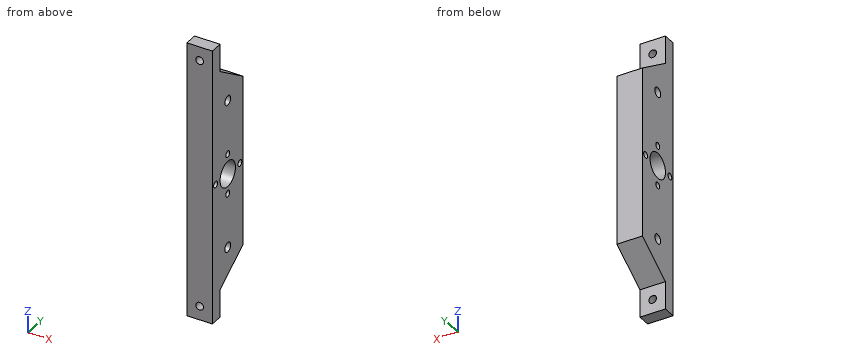
```python
from build123d import *

# Parameters (mm, degrees)
SKETCH2_W               = 380
SKETCH2_H               = 40
SKETCH2_R               = 10
SKETCH2_R_2             = 3.75
BOSS_EXTRUDE2_DEPTH     = 20
CUT_EXTRUDE1_DEPTH      = 100
CUT_EXTRUDE2_DEPTH      = 301.779846116
CUT_EXTRUDE2_DEPTH_BACK = 301.779846116
SKETCH5_R               = 3.023423491
SKETCH8_R               = 2.5
CUT_EXTRUDE3_DEPTH      = 302.941245658


with BuildPart() as part:
    # Sketch2 → Boss-Extrude2 (new body)
    with BuildSketch(Plane(origin=(0, 0, 0), x_dir=(0, 0, -1), z_dir=(1, 0, 0))):
        with Locations((190, 20)):
            Rectangle(SKETCH2_W, SKETCH2_H)
        with Locations((190, 20)):
            Circle(SKETCH2_R, mode=Mode.SUBTRACT)
        with Locations((131.63, 20)):
            Circle(SKETCH2_R_2, mode=Mode.SUBTRACT)
        with Locations((248.37, 20)):
            Circle(SKETCH2_R_2, mode=Mode.SUBTRACT)
    extrude(amount=BOSS_EXTRUDE2_DEPTH)

    # Sketch4 → Cut-Extrude1 (cut)
    with BuildSketch(Plane(origin=(20, 0, 0), x_dir=(0, 0, -1), z_dir=(1, 0, 0))):
        Polygon((123.129236316, 40), (0, 40), (0, 0), (81.389022591, 0), (81.389022591, 10), (103.1360247, 10), align=None)
        Polygon((298.610977409, 10), (298.610977409, 0), (380, 0), (380, 40), (256.870763684, 40), (276.8639753, 10), align=None)
    extrude(amount=-CUT_EXTRUDE1_DEPTH, mode=Mode.SUBTRACT)

    # Sketch5 → Cut-Extrude2 (cut, two sides: drawn at the far end of the back side and taken through both)
    with BuildSketch(Plane(origin=(0, 10, 0), x_dir=(1, 0, 0), z_dir=(0, 1, 0)).offset(-CUT_EXTRUDE2_DEPTH_BACK)):
        with Locations(Location((10, 92.262523645, 0), (0, 0, 270))):
            Circle(SKETCH5_R)
        with Locations(Location((10, 287.737476355, 0), (0, 0, 90))):
            Circle(SKETCH5_R)
    extrude(amount=CUT_EXTRUDE2_DEPTH + CUT_EXTRUDE2_DEPTH_BACK, mode=Mode.SUBTRACT)

    # Sketch8 → Cut-Extrude3 (cut, through all)
    with BuildSketch(Plane(origin=(20, 0, 0), x_dir=(0, 0, -1), z_dir=(1, 0, 0))):
        with Locations((190, 35.7650867)):
            Circle(SKETCH8_R)
        with Locations(Location((190, 4.2349133, 0), (0, 0, 180))):
            Circle(SKETCH8_R)
        with Locations((174.23, 20)):
            Circle(SKETCH8_R)
        with Locations(Location((205.77, 20, 0), (0, 0, 180))):
            Circle(SKETCH8_R)
    extrude(amount=-CUT_EXTRUDE3_DEPTH, mode=Mode.SUBTRACT)


solid = part.part
```
Input: part model. Units: mm. Frame: model coordinates. Coordinates: 2 decimals unless noted, no trailing zeros. Loops run counter-clockwise (first coordinate to the right, second up) from the corner with the lowest first, then second, coordinate; pieces in that order, holes last. Notation, with made-up numbers: (33.25, 5.25) - (82.25, 5.25) arc R29 ccw to (82.25, 29.25) - close; hole circle Ø11 at (56.5, 64.25). An arc over 180 degrees is marked (long way). Answer in a Markdown table with one row per item.
(1) Cut plane B-B on y = 14. Output: boundary loops of the cut face in (x, z).
Model answer:
| item | result |
|---|---|
| outline | (0, -274.2) - (20, -274.2) - (20, -198) - (0, -198) - close; (0, -182) - (20, -182) - (20, -105.8) - (0, -105.8) - close |
(2) Material intervals for L1, parallel to Y at x = 15.5, z = -190; L2, parallel to Y at x = 4.5, z = -131.63; L3, parallel to Y at x = 7.5, z = -174.23, sorted ascending. Write a range as from..to.
Model answer:
| item | result |
|---|---|
| L1 | y = 0..1.73, 6.73..10, 30..33.27, 38.27..40 |
| L2 | y = 0..16.25, 23.75..40 |
| L3 | y = 0..17.5, 22.5..40 |
(3) Pin query (flat end, axial travel): P1, Ø3.5, axis at x = 10, z = -287.74, coming from the +Y side; P2, Ø10, axis at x = 6.5, z = -290, coming from the +Y side; P3, Ø10, axis at x = 13, y = 31.5, coming from the +Z side. Return the tip coordinate at first contact, or that it passes through.
Model answer:
| item | result |
|---|---|
| P1 | passes through |
| P2 | stops at y = 10 |
| P3 | stops at z = -114.13 |
(4) Cut plane C-C on z = -190. Output: boundary loops of the cut face in (x, y), plus the area to 3 significant figures.
Model answer:
| item | result |
|---|---|
| outline | (0, 0) - (20, 0) - (20, 1.73) - (0, 1.73) - close; (0, 6.73) - (20, 6.73) - (20, 10) - (0, 10) - close; (0, 30) - (20, 30) - (20, 33.27) - (0, 33.27) - close; (0, 38.27) - (20, 38.27) - (20, 40) - (0, 40) - close |
| area | 200 mm² |
(5) Cut plane A-A on z = -131.63. Output: boundary loops of the cut face in (x, y), plus the area to 3 significant figures.
Model answer:
| item | result |
|---|---|
| outline | (0, 0) - (20, 0) - (20, 16.25) - (0, 16.25) - close; (0, 23.75) - (20, 23.75) - (20, 40) - (0, 40) - close |
| area | 650 mm² |
(6) Cut plane D-D on x = 15.5. Output: boundary loops of the cut face in (y, z).
Model answer:
| item | result |
|---|---|
| outline | (0, -298.61) - (10, -298.61) - (10, -276.86) - (40, -256.87) - (40, -123.13) - (10, -103.14) - (10, -81.39) - (0, -81.39) - close; hole circle Ø5 at (4.23, -190); hole circle Ø20 at (20, -190); hole circle Ø7.5 at (20, -248.37); hole circle Ø7.5 at (20, -131.63); hole circle Ø5 at (20, -205.77); hole circle Ø5 at (20, -174.23); hole circle Ø5 at (35.77, -190) |
